Check sheet for the modelled part. Datum: model origin and axes. Units: mm. A direction names the side the tool comes from. Round coordinates to 2 decimals unless told otherwise and drop trailing zeros. Loops run counter-clockwise (first coordinate to the right, second up) from the corner with the lowest first, then second, coordinate; pieces in that order, holes last. Notation, with made-up numbers: (36, -4) -> (49, -4) arc R23 cw to (49, 22) -> close; hole circle Ø8 at (80.5, 48.25). An arc over 180 degrees is marked (long way). Use one line per item in the form item = value. Start each with the question number.
(1) Material ranges on probe 1 along X at (y, z) = (0, 2.25); probe 2 along Y at (x, z) = (40, 1.5); probe 3 along X at (y, z) = (2, 9.75), recorded low to high. Write a range as [from, to].
(2) Go/stop test with flat-tipped pins: pin 1 (2 mm diameter, centred on x = 50, y = -7.5, fed in from -Z); pin 2 (4 mm diameter, centred on x = 39, y = 0, fed in from +Z); pin 3 (3 mm diameter, centred on x = 40, y = 0, fed in from +Z) (3 decimals); pin 4 (2.5 mm diameter, centred on x = 51.5, z = 2, fed in from -Y). Record where each tip stops, or that it passes through.
(3) Sectioned sample at B-B (x = 40). Record the cut outline in (y, z).
(4) Sectioned sample at C-C (z = 3). Record the cut outline in (x, y), and give its area (3 significant figures).
(5) Sectioned sample at D-D (y = -7.25). Record the cut outline in (x, z).
(6) Draft check along Y on faces 1 (the flat face through (-52, -8, 5)), 2 (the cylindrical face through (-38.383, -0.67, 3.451)), 3 (the flat face through (-52, -5.9, 2)). Enter one of: released by +Y, released by -Y, zero draft, split by the parting line, or undercut.
(7) Set-up check for faces 4 (the flat face through (-48.43, -7.98, 2.46)), 5 (the cylindrical face through (-70, 0, 7)), 6 (the flat face through (36.43, 2.02, 11.06)): record each of +Z, -Z, +X, -X, +Y, -Y from which the full face is reachable in a straight line by a thin tool's end or side.
(8) Sectioned sample at A-A (z = 12.5). Record the cut outline in (x, y).
from build123d import *

# Parameters (mm, degrees)
SKETCH_R        = 1.75
PAD_DEPTH       = 15
POCKET_DEPTH    = 8
POCKET001_DEPTH = 5


with BuildPart() as part:
    # Sketch → Pad (new body)
    with BuildSketch(Plane.XY):
        with BuildLine():
            ThreePointArc((-60.000035, 10), (-70, -1.7e-05), (-60, -10))
            Line((-60, -10), (60, -10))
            ThreePointArc((60, -10), (70, 1.5e-05), (59.999971, 10))
            Line((-60.000035, 10), (59.999971, 10))
        make_face()
        with Locations((40, 0)):
            Circle(SKETCH_R, mode=Mode.SUBTRACT)
        with Locations((-40, 0)):
            Circle(SKETCH_R, mode=Mode.SUBTRACT)
    extrude(amount=PAD_DEPTH)

    # Sketch001 → Pocket (cut)
    with BuildSketch(Plane.XY.offset(15)):
        Polygon((-42.367136, 4.1), (-37.632864, 4.1), (-35.265728, 0), (-37.632864, -4.1), (-42.367136, -4.1), (-44.734272, 0), align=None)
        Polygon((37.632864, 4.1), (42.367136, 4.1), (44.734272, 0), (42.367136, -4.1), (37.632864, -4.1), (35.265728, 0), align=None)
    extrude(amount=-POCKET_DEPTH, mode=Mode.SUBTRACT)

    # Sketch002 → Pocket001 (cut)
    with BuildSketch(Plane(origin=(0, 0, 0), x_dir=(1, 0, 0), z_dir=(0, 0, -1))):
        Polygon((-54.367136, 14.1), (-49.632864, 14.1), (-47.265728, 10), (-49.632864, 5.9), (-54.367136, 5.9), (-56.734272, 10), align=None)
        Polygon((49.632864, 14.1), (54.367136, 14.1), (56.734272, 10), (54.367136, 5.9), (49.632864, 5.9), (47.265728, 10), align=None)
    extrude(amount=-POCKET001_DEPTH, mode=Mode.SUBTRACT)


solid = part.part
Checks:
q1.probe_1 = [-70, -41.75], [-38.25, 38.25], [41.75, 70]
q1.probe_2 = [-10, -1.75], [1.75, 10]
q1.probe_3 = [-69.8, -43.58], [-36.42, 36.42], [43.58, 69.8]
q2.pin_1 = 5
q2.pin_2 = 7
q2.pin_3 = through
q2.pin_4 = -5.9
q3.outline = (-10, 0) -> (-1.75, 0) -> (-1.75, 7) -> (-4.1, 7) -> (-4.1, 15) -> (-10, 15) -> close; (1.75, 0) -> (10, 0) -> (10, 15) -> (4.1, 15) -> (4.1, 7) -> (1.75, 7) -> close
q4.outline = (-60, -10) -> (-56.73, -10) -> (-54.37, -5.9) -> (-49.63, -5.9) -> (-47.27, -10) -> (47.27, -10) -> (49.63, -5.9) -> (54.37, -5.9) -> (56.73, -10) -> (60, -10) arc R10 ccw to (60, 10) -> (-60, 10) arc R10 ccw to start; hole circle Ø3.5 at (-40, 0); hole circle Ø3.5 at (40, 0)
q4.area = 2,640 mm2
q5.outline = (-66.89, 0) -> (-55.15, 0) -> (-55.15, 5) -> (-48.85, 5) -> (-48.85, 0) -> (48.85, 0) -> (48.85, 5) -> (55.15, 5) -> (55.15, 0) -> (66.89, 0) -> (66.89, 15) -> (-66.89, 15) -> close
q6.face_1 = zero draft
q6.face_2 = undercut
q6.face_3 = released by -Y
q7.face_4 = -Z, -Y
q7.face_5 = +Z, -Z, -X
q7.face_6 = +Z
q8.outline = (-60, -10) -> (60, -10) arc R10 ccw to (60, 10) -> (-60, 10) arc R10 ccw to start; hole (-44.73, 0) -> (-42.37, -4.1) -> (-37.63, -4.1) -> (-35.27, 0) -> (-37.63, 4.1) -> (-42.37, 4.1) -> close; hole (35.27, 0) -> (37.63, -4.1) -> (42.37, -4.1) -> (44.73, 0) -> (42.37, 4.1) -> (37.63, 4.1) -> close
